Geometry check sheet. Reference: the model listing, model coordinates, mm. A direction names the side the tool comes from. Coordinates: 2 decimals unless noted, no trailing zeros. Loops run counter-clockwise (first coordinate to the right, second up) from the corner with the lowest first, then second, coordinate; pieces in that order, holes last. Notation, with made-up numbers: (-14.5, 52) -> (6.5, 52) arc R19 ccw to (6.5, 83) -> close; hole circle Ø11 at (50.5, 36.25). An arc over 180 degrees is marked (long way). Answer as a JSON object with one key per item and string values.
from build123d import *

# Parameters (mm, degrees)
F0_R          = 20.066
F1_DEPTH      = 30.226
F1_DEPTH_BACK = 30.226
F2_R          = 29.21
F2_R_2        = 20.066
F3_DEPTH      = 10.16
F4_R          = 29.21
F4_R_2        = 20.066
F5_DEPTH      = 10.16
F6_R          = 27.31135
F7_DEPTH      = 5.461
F8_R          = 27.31135
F9_DEPTH      = 5.461
F10_R         = 16.891
F11_DEPTH     = 75.312
F12_R         = 1.4732
F13_DEPTH     = 75.312
F16_DEPTH     = 49.277


with BuildPart() as f1:
    # F0 (on Right) → F1 (new body, two sides)
    with BuildSketch(Plane.YZ) as f1_sk:
        Circle(F0_R)
    extrude(amount=F1_DEPTH)
    extrude(f1_sk.sketch, amount=-F1_DEPTH_BACK)

    # F2 (on face) → F3 (join)
    with BuildSketch(Plane.YZ.offset(30.226)):
        Circle(F2_R)
        Circle(F2_R_2, mode=Mode.SUBTRACT)
        Circle(F2_R_2)
    extrude(amount=F3_DEPTH)

    # F4 (on face) → F5 (join)
    with BuildSketch(Plane(origin=(-30.226, 0, 0), x_dir=(0, -1, 0), z_dir=(-1, 0, 0))):
        Circle(F4_R)
        Circle(F4_R_2, mode=Mode.SUBTRACT)
        Circle(F4_R_2)
    extrude(amount=F5_DEPTH)

    # F6 (on face) → F7 (cut)
    with BuildSketch(Plane(origin=(-40.386, 0, 0), x_dir=(0, -1, 0), z_dir=(-1, 0, 0))):
        Circle(F6_R)
    extrude(amount=-F7_DEPTH, mode=Mode.SUBTRACT)

    # F8 (on face) → F9 (cut)
    with BuildSketch(Plane.YZ.offset(40.386)):
        Circle(F8_R)
    extrude(amount=-F9_DEPTH, mode=Mode.SUBTRACT)

    # F10 (on face) → F11 (cut, through all)
    with BuildSketch(Plane.YZ.offset(34.925)):
        Circle(F10_R)
    extrude(amount=-F11_DEPTH, mode=Mode.SUBTRACT)

    # F12 (on face) → F13 (cut, through all)
    with BuildSketch(Plane.YZ.offset(34.925)):
        with Locations((-21.7678, 12.573)):
            Circle(F12_R)
        with Locations((-12.573, 21.7678)):
            Circle(F12_R)
        with Locations((12.573, 21.7678)):
            Circle(F12_R)
        with Locations((21.7678, 12.573)):
            Circle(F12_R)
        with Locations((21.7678, -12.573)):
            Circle(F12_R)
        with Locations((12.573, -21.7678)):
            Circle(F12_R)
        with Locations((-12.573, -21.7678)):
            Circle(F12_R)
        with Locations((-21.7678, -12.573)):
            Circle(F12_R)
    extrude(amount=-F13_DEPTH, mode=Mode.SUBTRACT)

    # F15 (on offset) → F16 (cut, through all)
    with BuildSketch(Plane.XY.offset(20.066)):
        with BuildLine():
            Line((19.05, 30.226), (-19.05, 30.226))
            Line((-19.05, 30.226), (-19.05, 23.876))
            ThreePointArc((-19.05, 23.876), (-15.3302561211, 14.8957438789), (-6.35, 11.176))
            Line((-6.35, 11.176), (6.35, 11.176))
            ThreePointArc((6.35, 11.176), (15.3302561211, 14.8957438789), (19.05, 23.876))
            Line((19.05, 23.876), (19.05, 30.226))
        make_face()
        with BuildLine():
            Line((6.35, -11.176), (-6.35, -11.176))
            ThreePointArc((-6.35, -11.176), (-15.3302561211, -14.8957438789), (-19.05, -23.876))
            Line((-19.05, -23.876), (-19.05, -30.226))
            Line((-19.05, -30.226), (19.05, -30.226))
            Line((19.05, -30.226), (19.05, -23.876))
            ThreePointArc((19.05, -23.876), (15.3302561211, -14.8957438789), (6.35, -11.176))
        make_face()
    extrude(amount=-F16_DEPTH, mode=Mode.SUBTRACT)


solid = f1.part
1. Section check A-A, the plane x = 2. Record the boundary of the cut face in (y, z).
Evaluation:
{"outline": "(-11.18, -16.67) arc R20.07 ccw to (11.18, -16.67) -> (11.18, -12.67) arc R16.89 cw to (-11.18, -12.67) -> close; (-11.18, 12.67) arc R16.89 cw to (11.18, 12.67) -> (11.18, 16.67) arc R20.07 ccw to (-11.18, 16.67) -> close"}
2. Thickness scan on probe 1 along X at (y, z) = (-20, 11) (3 decimals); probe 2 along Y at (x, z) = (22, 0); probe 3 along Y at (x, z) = (-31, -12.5). Record the ranges inside material, lowest first. Write a range as from..to.
Evaluation:
{"probe 1": "x = -34.925..-30.226, 30.226..34.925", "probe 2": "y = -20.07..-16.89, 16.89..20.07", "probe 3": "y = -26.4..-23.24, -20.3..-11.36, 11.36..20.3, 23.24..26.4"}
3. Section check C-C, the plane z = 0. State how many separate pieces and enclosed holes the cut face has, then the cut area to 3 significant figures.
Evaluation:
{"separate pieces": "4", "enclosed holes": "0", "area": "431 mm^2"}
4. Depth check by flat-ended pin: P1, Ø1.2, axis at x = 0.5, z = 14, coming from the -Y side; P2, Ø4, axis at y = 21.77, z = 12.57, coming from the -X side (3 decimals); P3, Ø6, axis at x = 11, z = -19, coming from the -Y side; P4, Ø1.8, axis at y = -21.77, z = -12.57, coming from the -X side. Enter the tip coordinate at first touch or a pass-through.
Evaluation:
{"P1": "stops at y = -11.18", "P2": "stops at x = -34.925", "P3": "stops at y = -12.11", "P4": "passes through"}
5. Section check B-B, the plane y = 0. Record the boundary of the cut face in (x, z) (3 decimals), then the cut area to 3 significant figures.
Evaluation:
{"outline": "(-40.386, -29.21) -> (-30.226, -29.21) -> (-30.226, -20.066) -> (30.226, -20.066) -> (30.226, -29.21) -> (40.386, -29.21) -> (40.386, -27.311) -> (34.925, -27.311) -> (34.925, -16.891) -> (-34.925, -16.891) -> (-34.925, -27.311) -> (-40.386, -27.311) -> close; (-40.386, 27.311) -> (-34.925, 27.311) -> (-34.925, 16.891) -> (34.925, 16.891) -> (34.925, 27.311) -> (40.386, 27.311) -> (40.386, 29.21) -> (30.226, 29.21) -> (30.226, 20.066) -> (-30.226, 20.066) -> (-30.226, 29.21) -> (-40.386, 29.21) -> close", "area": "657 mm^2"}
6. Mould release check, pull along Z, two halves, no side actions. Record for faces 1 (the face through (40.386, 22, -17)), 2 (the face through (-35.23, 21.53, 19.74)), 3 (the face through (-32.54, -23.24, 12.64)), 4 (the face through (34.925, 12, 13)): released by +Z, released by -Z, zero draft, split by the parting line, or undercut.
Evaluation:
{"face 1": "zero draft", "face 2": "split by the parting line", "face 3": "undercut", "face 4": "undercut"}
7. Tool access check on faces 5 (the face through (17.11, -17.13, -1.16)), 6 (the face through (0, 11.176, -15)), 7 (the face through (37.69, -3.56, 27.08)), 8 (the face through (-30.226, 7, -19)), 9 (the face through (-34.925, -12, 13)). Record the directions out of +Z, -Z, +X, -X, +Y, -Y that give a thin tool (end or side, any length) a straight path to the whole face; none if there is none.
Evaluation:
{"face 5": "+Z, -Z, -Y", "face 6": "+Z, -Z, +Y", "face 7": "+X", "face 8": "none", "face 9": "-X"}
